```python
from build123d import *

# Parameters (mm, degrees)
F2_W      = 40
F2_H      = 40
F0_W      = 40
F0_H      = 40
F4_W      = 20
F4_H      = 20
F5_DEPTH  = 30
F6_W      = 20
F6_H      = 20
F7_DEPTH  = 30
F8_R      = 3
F9_DEPTH  = 10
F10_R     = 3
F11_DEPTH = 10
F12_R     = 3
F13_DEPTH = 4
F14_R     = 2.339203
F15_DEPTH = 4
F16_W     = 19
F16_H     = 20
F17_DEPTH = 54
F18_R     = 3
F19_DEPTH = 4
F20_R     = 3
F21_DEPTH = 10


with BuildPart() as f3:
    # F2 (on offset) → F3 section 0
    with BuildSketch(Plane.XY.offset(410)):
        with Locations((92.29407, 92.29407)):
            Rectangle(F2_W, F2_H)
    # F0 (on Top) → F3 section 1
    with BuildSketch(Plane.XY):
        with Locations((20, 20)):
            Rectangle(F0_W, F0_H)
    loft()

    # F4 (on Right) → F5 (cut)
    with BuildSketch(Plane.YZ):
        with Locations((20, 10)):
            Rectangle(F4_W, F4_H)
    extrude(amount=F5_DEPTH, mode=Mode.SUBTRACT)

    # F6 (on Front) → F7 (cut)
    with BuildSketch(Plane.XZ):
        with Locations((20, 10)):
            Rectangle(F6_W, F6_H)
    extrude(amount=-F7_DEPTH, mode=Mode.SUBTRACT)

    # F8 (on face) → F9 (cut)
    with BuildSketch(Plane(origin=(0, 0, 0), x_dir=(1, 0, 0), z_dir=(0, -0.984808, 0.173648))):
        with Locations((88.165338, 390.824912)):
            Circle(F8_R)
    extrude(amount=-F9_DEPTH, mode=Mode.SUBTRACT)

    # F10 (on face) → F11 (cut)
    with BuildSketch(Plane(origin=(0, 0, 0), x_dir=(0, -1, 0), z_dir=(-0.984808, 0, 0.173648))):
        with Locations((-88.165338, 390.824912)):
            Circle(F10_R)
    extrude(amount=-F11_DEPTH, mode=Mode.SUBTRACT)

    # F12 (on face) → F13 (cut)
    with BuildSketch(Plane(origin=(30, 0, 0), x_dir=(0, -1, 0), z_dir=(-1, 0, 0))):
        with Locations((-20, 10)):
            Circle(F12_R)
    extrude(amount=-F13_DEPTH, mode=Mode.SUBTRACT)

    # F14 (on face) → F15 (cut)
    with BuildSketch(Plane.XZ.offset(-30)):
        with Locations((20, 10)):
            Circle(F14_R)
    extrude(amount=-F15_DEPTH, mode=Mode.SUBTRACT)

    # F16 (on Front) → F17 (cut)
    with BuildSketch(Plane.XZ):
        with Locations((44.441441, 210)):
            Rectangle(F16_W, F16_H)
    extrude(amount=-F17_DEPTH, mode=Mode.SUBTRACT)

    # F18 (on face) → F19 (cut)
    with BuildSketch(Plane(origin=(53.941441, 0, 0), x_dir=(0, -1, 0), z_dir=(-1, 0, 0))):
        with Locations((-44, 210)):
            Circle(F18_R)
    extrude(amount=-F19_DEPTH, mode=Mode.SUBTRACT)

    # F20 (on face) → F21 (cut)
    with BuildSketch(Plane.XY.offset(410)):
        with Locations((92.29407, 92.29407)):
            Circle(F20_R)
    extrude(amount=-F21_DEPTH, mode=Mode.SUBTRACT)


solid = f3.part
```
The model under review builds one solid part; all positions refer to its coordinate system, in mm. A direction names the side the tool comes from. Coordinates: 2 decimals unless noted, no trailing zeros.
1) The part is to be moulded in two halves that separate along Y. For faces 1 (the face through (44, 54, 210)), 2 (the face through (87.77, 73.24, 386.96)), 3 (the face through (5, 5, 0)), 4 (the face through (6, 10, 10)), say which applies: pulls with the +Y half, pulls with the -Y half, needs draft (parallel to the pull), parting line crosses it, or undercut.
2) Clearance check with flat-ended pins moving along their axes: pin 1 Ø3.5 at (x, y) = (92.29, 92.29) entering from +Z; pin 2 Ø5 at (x, z) = (2.5, 14.5) entering from +Y; pin 3 Ø5 at (x, z) = (29.5, 171.5) entering from +Y. State where each tip first meets the part, or that it passes through.
3) Machinability: for faces 5 (the face through (96, 88, 410)), 6 (the face through (72.26, 86.78, 381.41)), 7 (the face through (46, 46, 220)), 8 (the face through (10, 6, 10)), 9 (the face through (15, 30, 10)), which of the approach directions +Z, -Z, +X, -X, +Y, -Y give a long, thin tool a straight path to every point of the face, cutting with its end or side? Answer none if there is none.
4) To check wall thickness, follow probe 1 along X at (y, z) = (34, 27.5); probe 2 along X at (y, z) = (86.5, 305); probe 3 along Y at (x, z) = (57.05, 210). State the ranges of each line that lie inside material, in increasing order.
Answer list:
1. face 1: pulls with the -Y half
1. face 2: undercut
1. face 3: needs draft
1. face 4: undercut
2. pin 1: stops at z = 400
2. pin 2: stops at y = 42.99
2. pin 3: stops at y = 70.63
3. face 5: +Z, +X, -X, +Y, -Y
3. face 6: none
3. face 7: -X, -Y
3. face 8: -Z, -Y
3. face 9: -Z, -X
4. probe 1: x = 4.85 to 44.85
4. probe 2: x = 53.78 to 93.78
4. probe 3: y = 37.03 to 41, 47 to 77.03
